Read the model definition and answer for the solid it produces. Units are mm, in the model's axes. A direction names the side the tool comes from. Coordinates: 2 decimals unless noted, no trailing zeros. Order: outer loops, then holes, each group sorted by start corner. A loop starts at its lowest first (then second) coordinate and runs counter-clockwise, first axis right, second up. Notation, with made-up numbers: M 5.25,7 L 54.25,7 A18 cw 54.25,20 Z; hole C -39.5,28 d2. An arc over 180 degrees is marked long. One line per question, with ' | ' between items. Start each with the question number.
1) A tool of negligible diameter and unlimited length cuts with its end or side. For faces 1 (the face through (-8.264, -5.24, 7.466)), 2 (the face through (3, 7, 20)), 3 (the face through (-3, 9, 11)), 4 (the face through (3, 7, 0)), from which of +Z, -Z, +X, -X, +Y, -Y can it reach the whole face along a straight path? Write none if from no direction.
2) The mould has two halves that part along Y. Classify faces 5 (the face through (-3, -9, 0)), 6 (the face through (9.96, -1.9, 20.57)), 7 (the face through (-8, -4.5, 9)), 8 (the face through (9.96, -3.07, -9.4)): +Y half, -Y half, draft (parallel to the pull), parting line (faces both ways), or undercut.
3) Find section B-B, the plane z = 10. Write down the section's boundary in (x, y), plus the area to 4 significant figures.
4) Find section C-C, the plane z = -6. Write down the section's boundary in (x, y), plus the area to 3 significant figures.
5) Find section D-D, the plane x = -5.5. Count the separate pieces of the cut face and the enclosed holes in it, plus the area to 3 significant figures.
6) Consider probe 1 along Y at (x, z) = (8.65, 26); probe 2 along Z at (x, y) = (-5.5, 11.5); probe 3 along Z at (x, y) = (-5.5, 5.9). Determine where each line is inside the solid, lowest interval first.
7) Given P1, Ø4, axis at x = 2, y = 10, coming from the +Z side; P2, Ø12, axis at x = -9, y = -0.5, coming from the -Z side; P3, Ø2, axis at x = -2.5, y = -9.5, coming from the +Z side, each flat-ended and moving along its own axis, determine where each tip first touches the part or whether it passes through.
8) Find section A-A, the plane y = -7.5. Write down the section's boundary in (x, z).
Autodesk Inventor part; units mm, degrees
ref_plane "YZ Plane" through (0, 0, 0) normal (1, 0, 0) x (0, 1, 0)
ref_plane "XZ Plane" through (0, 0, 0) normal (0, 1, 0) x (-1, 0, 0)
ref_plane "XY Plane" through (0, 0, 0) normal (0, 0, 1) x (1, 0, 0)
sketch "Sketch1" plane through (0, 0, 0) normal (0, 0, 1) x (1, 0, 0)
  line L0 (-12.5, 12.5) -> (12.5, 12.5)
  line L1 (12.5, 12.5) -> (12.5, -12.5)
  line L2 (12.5, -12.5) -> (-12.5, -12.5)
  line L3 (-12.5, -12.5) -> (-12.5, 12.5)
  point P0 (0, 0)
  point P1 (-12.5, 0)
  point P2 (0, 12.5)
  dimension "d0" = 25
  dimension "d1" = 25
extrude "Extrusion1" add sketch "Sketch1" along normal blind 20
sketch "Sketch2" plane through (0, 0, 20) normal (0, 0, 1) x (1, 0, 0)
  line L0 (-12.5, -6) -> (7.5, -6)
  line L1 (7.5, -6) -> (7.5, 6)
  line L2 (7.5, 6) -> (-12.5, 6)
  line L3 (-12.5, 6) -> (-12.5, -6)
  line L4 (-12.5, 12.5) -> (-12.5, -12.5)
  line L5 (12.5, -12.5) -> (12.5, 12.5)
  point P0 (0, 0)
  point P1 (7.5, 0)
  point P2 (12.5, 0)
  dimension "d4" = 12
  dimension "d5" = 5
extrude "Extrusion2" cut sketch "Sketch2" against normal through all
sketch "Sketch3" plane through (-12.5, -12.5, 0) normal (0, -1, 0) x (1, 0, 0)
  line L0 (0, 0) -> (0, 20)
  point P0 (12.5, 0)
  point P1 (7, 10)
  point P2 (0, 10)
  dimension "d8" = 7
hole "Hole1" at (-5.5, -12.5, 10) direction (0, 1, 0) diameter 5 end through all
sketch "Sketch4" plane through (-12.5, 12.5, 0) normal (0, 1, 0) x (1, 0, 0)
  line L0 (25, -23) -> (0, -23)
  line L1 (0, -23) -> (0, -20)
  line L2 (0, -20) -> (25, -20)
  line L3 (25, -20) -> (25, -23)
  line L4 (25, -20) -> (0, -20)
  line L5 (0, 0) -> (0, -20)
  line L6 (25, 0) -> (25, -20)
  line L7 (25, 0) -> (0, 0)
  line L8 (0, 0) -> (0, 3)
  line L9 (0, 3) -> (25, 3)
  line L10 (25, 3) -> (25, 0)
  line L11 (25, 0) -> (0, 0)
  point P0 (12.5, 0)
  dimension "d16" = 3
extrude "Extrusion3" add sketch "Sketch4" against normal blind 3 contours L0 L1 L2 L3 | L7 L8 L9 L10
sketch "Sketch7" plane through (12.5, -12.5, 20) normal (1, 0, 0) x (0, 0, -1)
  line L0 (-10, 0) -> (-10, 10)
  line L1 (-10, 10) -> (30, 10)
  line L2 (30, 10) -> (30, 0)
  line L3 (20, 0) -> (0, 0)
  line L4 (20, 0) -> (20, 22)
  line L5 (0, 0) -> (0, 22)
  circle A0 centre (26, 5) radius 2.25
  circle A1 centre (-6, 5) radius 2.25
  line L6 (20, 0) -> (0, 0)
  line L7 (-10, 0) -> (32.446, 0)
  point P0 (20, 12.5)
  point P1 (30, 5)
  point P2 (20, 10)
  point P3 (0, 10)
  point P4 (20, 0)
  point P5 (0, 0)
  dimension "d30" = 10
  dimension "d31" = 10
  dimension "d32" = 4.5
  dimension "d33" = 4
  dimension "d34" = 4
  dimension "d50" = 10
  dimension "d51" = 0
extrude "Extrusion5" add sketch "Sketch7" against normal up to surface (5 mm away) contours L0 L1 L5 L7 | L4 L1 L2 L7
sketch "Sketch6" plane through (-12.5, 12.5, 23) normal (0, 1, 0) x (1, 0, 0)
  circle A0 centre (7, 13) radius 2.5
  circle A1 centre (7, 13) radius 1.5
  point P0 (12.5, 23)
  dimension "d26" = 3
extrude "Extrusion4" add sketch "Sketch6" against normal blind 2
sketch "Sketch8" plane through (-12.5, 12.5, 23) normal (0, 1, 0) x (1, 0, 0)
  circle A0 centre (7, 13) radius 1.5
  circle A1 centre (7, 13) radius 3.75
  point P0 (12.5, 23)
  dimension "d37" = 7.5
extrude "Extrusion6" add sketch "Sketch8" against normal up to surface (25 mm away)
sketch "Sketch9" plane through (-12.5, 12.5, 23) normal (0, 0, 1) x (1, 0, 0)
  line L0 (0, -8) -> (20, -8)
  line L1 (20, -8) -> (20, -17)
  line L2 (20, -17) -> (0, -17)
  line L3 (0, -17) -> (0, -8)
  line L4 (0, -18.5) -> (0, -25)
  line L5 (20, -6.5) -> (20, -18.5)
  line L6 (0, -6.5) -> (20, -6.5)
  line L7 (20, -18.5) -> (0, -18.5)
  point P0 (12.5, -12.5)
  point P1 (20, -15)
  dimension "d40" = 1.5
  dimension "d41" = 1.5
extrude "Extrusion7" cut sketch "Sketch9" against normal through all
move faces "Move2" translate (0, 1.5, 0) faces at (7, 12.5, 10)
fillet "Fillet2" radius 2 6 edges at (10, -2.5, 20) (10, -2.5, 30) (10, -12.5, 30) (10, -12.5, -10) (10, -2.5, -10) (10, -2.5, 0)
sketch "Sketch11" plane through (-12.5, 14, 23) normal (0, 1, 0) x (1, 0, 0)
  circle A0 centre (7, 13) radius 1.5
  point P0 (12.5, 23)
hole "Hole3" at (-5.5, 14, 10) direction (0, -1, 0) diameter 5 end through all counterbore diameter 11 counterbore depth 5
equation "\"d30\" = d31"
properties part number "10-03-024"
Report:
1) face 1: none | face 2: +Z, +X, -X | face 3: +Y | face 4: -Z, +X, -X
2) face 5: draft | face 6: undercut | face 7: undercut | face 8: +Y half
3) outline: M -12.5,-12.5 L -8,-12.5 L -8,-4.5 L -9.25,-4.5 L -9.25,-6 L -12.5,-6 Z; M -12.5,6 L -9.25,6 L -9.25,4.5 L -8,4.5 L -8,9 L -11,9 L -11,14 L -12.5,14 Z; M -3,-12.5 L 12.5,-12.5 L 12.5,14 L 0,14 L 0,9 L -3,9 L -3,4.5 L -1.75,4.5 L -1.75,6 L 7.5,6 L 7.5,-6 L -1.75,-6 L -1.75,-4.5 L -3,-4.5 Z | area: 327.5 mm^2
4) outline: M 7.5,-12.5 L 12.5,-12.5 L 12.5,-9.75 L 7.5,-9.75 Z; M 7.5,-5.25 L 12.5,-5.25 L 12.5,-2.5 L 7.5,-2.5 Z | area: 27.5 mm^2
5) separate pieces: 4 | enclosed holes: 0 | area: 222 mm^2
6) probe 1: y = -12.5 to -9.75, -5.25 to -2.5 | probe 2: z = -3 to 4.5, 15.5 to 23 | probe 3: z = 6.25 to 7.5, 12.5 to 13.75
7) P1: stops at z = 23 | P2: stops at z = 0 | P3: stops at z = 20
8) outline: M -12.5,0 L 7.5,0 L 7.5,-3.75 L 12.5,-3.75 L 12.5,23.75 L 7.5,23.75 L 7.5,20 L -12.5,20 Z; M 7.5,-10 L 12.5,-10 L 12.5,-8.25 L 7.5,-8.25 Z; M 7.5,28.25 L 12.5,28.25 L 12.5,30 L 7.5,30 Z; hole C -5.5,10 d5
